Read the model definition and answer for the solid it produces. Units are mm, in the model's axes. Face numbers are marked on the shaded views. A direction names the side the tool comes from. Coordinates: 2 decimals unless noted, no trailing zeros. Write each loop counter-clockwise with the first axis right and the second up, starting at its lowest first coordinate (ties: lowest second). Pieces come first, ordered by that corner, then holes. Notation, with made-up numbers: (-5, 76.5) -> (20, 76.5) arc R6 cw to (20, 85.5) -> close; hole circle Ø7 at (-3, 13.25). An arc over 180 degrees is marked (long way). Use CSV: the item, a comma, the result in double quotes.
from build123d import *

# Parameters (mm, degrees)
SKETCH1_R           = 26.15
SKETCH1_R_2         = 2
SKETCH1_R_3         = 2.5
BOSS_EXTRUDE1_DEPTH = 30
BOSS_EXTRUDE2_START = -7
BOSS_EXTRUDE2_DEPTH = 16
CHAMFER1_SIZE       = 1.5
CUT_EXTRUDE1_DEPTH  = 90


with BuildPart() as part:
    # Sketch1 → Boss-Extrude1 (new body)
    with BuildSketch(Plane.XY):
        with BuildLine():
            Line((100, 15), (100, -15))
            Line((100, -15), (7.109450059, -34.270332941))
            ThreePointArc((7.109450059, -34.270332941), (-35, 0), (7.109450059, 34.270332941))
            Line((7.109450059, 34.270332941), (100, 15))
        make_face()
        Circle(SKETCH1_R, mode=Mode.SUBTRACT)
        with Locations((59, 0)):
            Circle(SKETCH1_R_2, mode=Mode.SUBTRACT)
        with Locations((78.6, 0)):
            Circle(SKETCH1_R_3, mode=Mode.SUBTRACT)
        with Locations((33, 0)):
            Circle(SKETCH1_R_2, mode=Mode.SUBTRACT)
    extrude(amount=BOSS_EXTRUDE1_DEPTH)

    # Sketch2 → Boss-Extrude2 (add)
    with BuildSketch(Plane.XY.offset(30).offset(BOSS_EXTRUDE2_START)):
        with BuildLine():
            Line((18.10386699, 12.5), (22.968946428, 12.5))
            ThreePointArc((22.968946428, 12.5), (-26.15, 0), (22.968946428, -12.5))
            Line((22.968946428, -12.5), (18.10386699, -12.5))
            ThreePointArc((18.10386699, -12.5), (-22, 0), (18.10386699, 12.5))
        make_face()
    extrude(amount=-BOSS_EXTRUDE2_DEPTH)

    # Chamfer1
    chamfer1_edges = [part.edges().sort_by_distance(p)[0] for p in [
        (-26.15, 0, 0),
        (-26.15, 0, 30),
        (53.554725029, -24.63516647, 30),
        (53.554725029, 24.63516647, 30),
        (53.554725029, -24.63516647, 0),
        (-35, 0, 0),
        (53.554725029, 24.63516647, 0),
        (-35, 0, 30),
    ]]
    chamfer(chamfer1_edges, length=CHAMFER1_SIZE)

    # Sketch3 → Cut-Extrude1 (cut)
    with BuildSketch(Plane(origin=(100, 0, 0), x_dir=(0, 0, -1), z_dir=(1, 0, 0))):
        with BuildLine():
            Line((-12.197056275, 4.5), (-17.802943725, 4.5))
            Line((-17.802943725, 4.5), (-19.710050506, 6.407106781))
            Line((-19.710050506, 6.407106781), (-19.710050506, 7.7))
            Line((-19.710050506, 7.7), (-18.482842712, 7.7))
            ThreePointArc((-18.482842712, 7.7), (-17.83612704, 8.132121597), (-17.987867966, 8.894974747))
            Line((-17.987867966, 8.894974747), (-19.387867966, 10.294974747))
            Line((-19.387867966, 10.294974747), (-25.294974747, 10.294974747))
            Line((-25.294974747, 10.294974747), (-25.294974747, 4.387867966))
            Line((-25.294974747, 4.387867966), (-23.894974747, 2.987867966))
            ThreePointArc((-23.894974747, 2.987867966), (-23.132121597, 2.83612704), (-22.7, 3.482842712))
            Line((-22.7, 3.482842712), (-22.7, 4.710050506))
            Line((-22.7, 4.710050506), (-21.407106781, 4.710050506))
            Line((-21.407106781, 4.710050506), (-19.5, 2.802943725))
            Line((-19.5, 2.802943725), (-19.5, -2.802943725))
            Line((-19.5, -2.802943725), (-21.407106781, -4.710050506))
            Line((-21.407106781, -4.710050506), (-22.7, -4.710050506))
            Line((-22.7, -4.710050506), (-22.7, -3.482842712))
            ThreePointArc((-22.7, -3.482842712), (-23.132121597, -2.83612704), (-23.894974747, -2.987867966))
            Line((-23.894974747, -2.987867966), (-25.294974747, -4.387867966))
            Line((-25.294974747, -4.387867966), (-25.294974747, -10.294974747))
            Line((-25.294974747, -10.294974747), (-19.387867966, -10.294974747))
            Line((-19.387867966, -10.294974747), (-17.987867966, -8.894974747))
            ThreePointArc((-17.987867966, -8.894974747), (-17.83612704, -8.132121597), (-18.482842712, -7.7))
            Line((-18.482842712, -7.7), (-19.710050506, -7.7))
            Line((-19.710050506, -7.7), (-19.710050506, -6.407106781))
            Line((-19.710050506, -6.407106781), (-17.802943725, -4.5))
            Line((-17.802943725, -4.5), (-12.197056275, -4.5))
            Line((-12.197056275, -4.5), (-10.289949494, -6.407106781))
            Line((-10.289949494, -6.407106781), (-10.289949494, -7.7))
            Line((-10.289949494, -7.7), (-11.517157288, -7.7))
            ThreePointArc((-11.517157288, -7.7), (-12.16387296, -8.132121597), (-12.012132034, -8.894974747))
            Line((-12.012132034, -8.894974747), (-10.612132034, -10.294974747))
            Line((-10.612132034, -10.294974747), (-4.705025253, -10.294974747))
            Line((-4.705025253, -10.294974747), (-4.705025253, -4.387867966))
            Line((-4.705025253, -4.387867966), (-6.105025253, -2.987867966))
            ThreePointArc((-6.105025253, -2.987867966), (-6.867878403, -2.83612704), (-7.3, -3.482842712))
            Line((-7.3, -3.482842712), (-7.3, -4.710050506))
            Line((-7.3, -4.710050506), (-8.592893219, -4.710050506))
            Line((-8.592893219, -4.710050506), (-10.5, -2.802943725))
            Line((-10.5, -2.802943725), (-10.5, 2.802943725))
            Line((-10.5, 2.802943725), (-8.592893219, 4.710050506))
            Line((-8.592893219, 4.710050506), (-7.3, 4.710050506))
            Line((-7.3, 4.710050506), (-7.3, 3.482842712))
            ThreePointArc((-7.3, 3.482842712), (-6.867878403, 2.83612704), (-6.105025253, 2.987867966))
            Line((-6.105025253, 2.987867966), (-4.705025253, 4.387867966))
            Line((-4.705025253, 4.387867966), (-4.705025253, 10.294974747))
            Line((-4.705025253, 10.294974747), (-10.612132034, 10.294974747))
            Line((-10.612132034, 10.294974747), (-12.012132034, 8.894974747))
            ThreePointArc((-12.012132034, 8.894974747), (-12.16387296, 8.132121597), (-11.517157288, 7.7))
            Line((-11.517157288, 7.7), (-10.289949494, 7.7))
            Line((-10.289949494, 7.7), (-10.289949494, 6.407106781))
            Line((-10.289949494, 6.407106781), (-12.197056275, 4.5))
        make_face()
    extrude(amount=-CUT_EXTRUDE1_DEPTH, mode=Mode.SUBTRACT)


solid = part.part
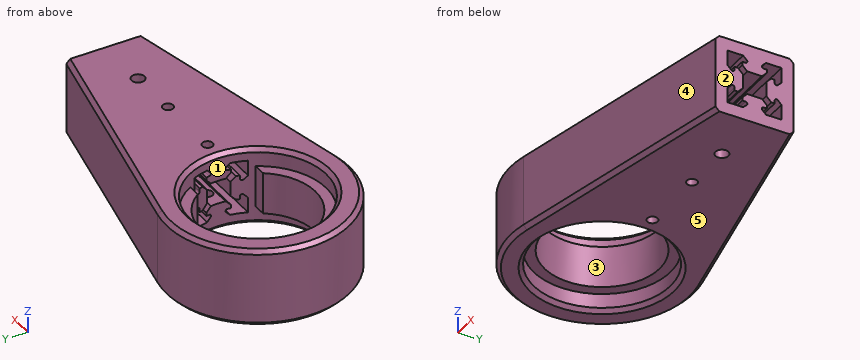
1. A cutting plane is placed at B-B (y = 0). Give the number of separate pieces and of enclosed holes in the cut face, and give its area (3 significant figures).
Solutions:
separate pieces,"9"
enclosed holes,"0"
area,"1,600 mm^2"
2. For a pull along Y with two mould halves and no side action, classify the marked faces 3, 4 and 5 as pulls with the +Y half, pulls with the -Y half, needs draft (parallel to the pull), parting line crosses it, or undercut.
Solutions:
face 3,"undercut"
face 4,"pulls with the -Y half"
face 5,"needs draft"
3. A tool of negligible diameter and unlimited length cuts with its end or side. For the marked faces 1 and 2, from which of +Z, -Z, +X, -X, +Y, -Y can it reach the whole face along a straight path? Write none if from no direction.
Solutions:
face 1,"none"
face 2,"+Z, -Z, +X, +Y, -Y"
4. A cutting plane is placed at C-C (z = 13.75). Give the vertices of the cut face in (x, y).
Solutions:
outline,"(7.11, -34.27) -> (100, -15) -> (100, -4.5) -> (25.76, -4.5) arc R26.15 cw to (22.97, -12.5) -> (18.1, -12.5) arc R22 cw (long way) to (18.1, 12.5) -> (22.97, 12.5) arc R26.15 cw to (25.76, 4.5) -> (100, 4.5) -> (100, 15) -> (7.11, 34.27) arc R35 ccw (long way) to start"
5. Find the intervals of material crossed by line 1 along X through (y, z) = (0, 4); line 2 along Y through (x, z) = (0, 12); line 3 along Y through (x, z) = (45, 5), in increasing order.
Solutions:
line 1,"x = -35 to -26.15, 26.15 to 31, 35 to 57, 61 to 76.1, 81.1 to 100"
line 2,"y = -35 to -22, 22 to 35"
line 3,"y = -26.41 to -10.29, -4.09 to 4.09, 10.29 to 26.41"
6. Each of these flat-tipped pins is pushed along its axis until it touches: pin 1 Ø4.5 at (x, z) = (52.5, 21.5) entering from -Y; pin 2 Ø1 at (x, z) = (48, 19) entering from +Y; pin 3 Ø4.5 at (x, z) = (74, 15) entering from -Y; pin 4 Ø8 at (x, y) = (5.5, 13) entering from -Z. Where does it stop, or does it pass through?
Solutions:
pin 1,"stops at y = -25.32"
pin 2,"stops at y = 25.89"
pin 3,"stops at y = -20.86"
pin 4,"passes through"
7. A cutting plane is placed at A-A (x = 0). Give the vertices of the cut face in (y, z), and give its area (3 significant figures).
Solutions:
outline,"(-35, 1.5) -> (-33.5, 0) -> (-27.65, 0) -> (-26.15, 1.5) -> (-26.15, 7) -> (-22, 7) -> (-22, 23) -> (-26.15, 23) -> (-26.15, 28.5) -> (-27.65, 30) -> (-33.5, 30) -> (-35, 28.5) -> close; (22, 7) -> (26.15, 7) -> (26.15, 1.5) -> (27.65, 0) -> (33.5, 0) -> (35, 1.5) -> (35, 28.5) -> (33.5, 30) -> (27.65, 30) -> (26.15, 28.5) -> (26.15, 23) -> (22, 23) -> close"
area,"655 mm^2"
